Part model, mm, in its own coordinate system. Face numbers are marked on the shaded views. A direction names the side the tool comes from. Give positions to 0.01 mm unless a question says otherwise; leave off trailing zeros. Order: outer loops, then holes, each group sorted by start corner. A loop starts at its lowest first (then second) coordinate and runs counter-clockwise, first axis right, second up. Notation, with made-up numbers: M 46,-36 L 65,-36 A11 cw 65,-28 Z; hole C 67,79.5 d10. An arc over 180 degrees is marked long. Write each question's results on one line, items separated by ' | '. Start each with the question number.
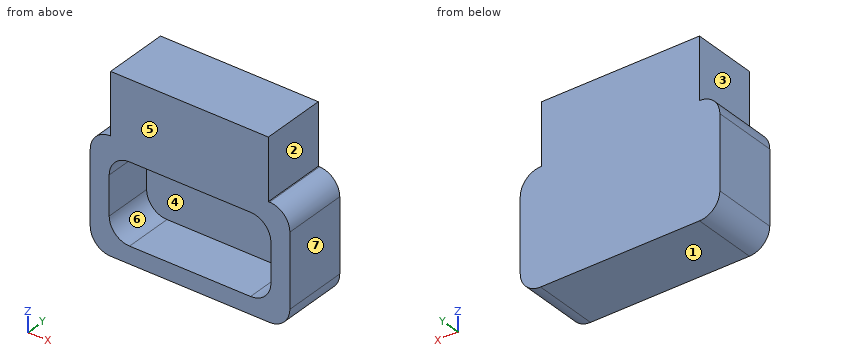
from build123d import *

# Parameters (mm, degrees)
F1_DEPTH = 19.05
F2_DEPTH = 5.08
F0_W     = 49.223448
F0_H     = 19.05
F3_DEPTH = 20.32


with BuildPart() as f1:
    # F0 (on Front) → F1 (new body)
    with BuildSketch(Plane.XZ):
        with BuildLine():
            Line((24.436552, 17.736208), (-24.786896, 17.736208))
            ThreePointArc((-24.786896, 17.736208), (-29.277025, 15.876336), (-31.136896, 11.386208))
            Line((-31.136896, 11.386208), (-31.136896, -11.386208))
            ThreePointArc((-31.136896, -11.386208), (-29.277025, -15.876336), (-24.786896, -17.736208))
            Line((-24.786896, -17.736208), (24.786896, -17.736208))
            ThreePointArc((24.786896, -17.736208), (29.277025, -15.876336), (31.136896, -11.386208))
            Line((31.136896, -11.386208), (31.136896, 11.386208))
            ThreePointArc((31.136896, 11.386208), (29.277025, 15.876336), (24.786896, 17.736208))
            Line((24.786896, 17.736208), (24.436552, 17.736208))
        make_face()
        with BuildLine():
            ThreePointArc((-25.224827, 6.065345), (-23.364955, 10.555473), (-18.874827, 12.415345))
            Line((-18.874827, 12.415345), (18.874827, 12.415345))
            ThreePointArc((18.874827, 12.415345), (23.364955, 10.555473), (25.224827, 6.065345))
            Line((25.224827, 6.065345), (25.224827, -6.065345))
            ThreePointArc((25.224827, -6.065345), (23.364955, -10.555473), (18.874827, -12.415345))
            Line((18.874827, -12.415345), (-18.874827, -12.415345))
            ThreePointArc((-18.874827, -12.415345), (-23.364955, -10.555473), (-25.224827, -6.065345))
            Line((-25.224827, -6.065345), (-25.224827, 6.065345))
        make_face(mode=Mode.SUBTRACT)
    extrude(amount=F1_DEPTH)

    # F0 (on Front) → F2 (join)
    with BuildSketch(Plane.XZ):
        with BuildLine():
            Line((18.874827, 12.415345), (-18.874827, 12.415345))
            ThreePointArc((-18.874827, 12.415345), (-23.364955, 10.555473), (-25.224827, 6.065345))
            Line((-25.224827, 6.065345), (-25.224827, -6.065345))
            ThreePointArc((-25.224827, -6.065345), (-23.364955, -10.555473), (-18.874827, -12.415345))
            Line((-18.874827, -12.415345), (18.874827, -12.415345))
            ThreePointArc((18.874827, -12.415345), (23.364955, -10.555473), (25.224827, -6.065345))
            Line((25.224827, -6.065345), (25.224827, 6.065345))
            ThreePointArc((25.224827, 6.065345), (23.364955, 10.555473), (18.874827, 12.415345))
        make_face()
    extrude(amount=F2_DEPTH)

    # F0 (on Front) → F3 (join)
    with BuildSketch(Plane.XZ):
        with Locations((-0.175172, 27.261208)):
            Rectangle(F0_W, F0_H)
        with BuildLine():
            Line((24.436552, 17.736208), (-24.786896, 17.736208))
            ThreePointArc((-24.786896, 17.736208), (-29.277025, 15.876336), (-31.136896, 11.386208))
            Line((-31.136896, 11.386208), (-31.136896, -11.386208))
            ThreePointArc((-31.136896, -11.386208), (-29.277025, -15.876336), (-24.786896, -17.736208))
            Line((-24.786896, -17.736208), (24.786896, -17.736208))
            ThreePointArc((24.786896, -17.736208), (29.277025, -15.876336), (31.136896, -11.386208))
            Line((31.136896, -11.386208), (31.136896, 11.386208))
            ThreePointArc((31.136896, 11.386208), (29.277025, 15.876336), (24.786896, 17.736208))
            Line((24.786896, 17.736208), (24.436552, 17.736208))
        make_face()
        with BuildLine():
            ThreePointArc((-25.224827, 6.065345), (-23.364955, 10.555473), (-18.874827, 12.415345))
            Line((-18.874827, 12.415345), (18.874827, 12.415345))
            ThreePointArc((18.874827, 12.415345), (23.364955, 10.555473), (25.224827, 6.065345))
            Line((25.224827, 6.065345), (25.224827, -6.065345))
            ThreePointArc((25.224827, -6.065345), (23.364955, -10.555473), (18.874827, -12.415345))
            Line((18.874827, -12.415345), (-18.874827, -12.415345))
            ThreePointArc((-18.874827, -12.415345), (-23.364955, -10.555473), (-25.224827, -6.065345))
            Line((-25.224827, -6.065345), (-25.224827, 6.065345))
        make_face(mode=Mode.SUBTRACT)
    extrude(amount=F3_DEPTH)


solid = f1.part
(1) Drop flat-ended pins along their axis: P1, Ø8, axis at x = 11.5, z = -7.5, coming from the -Y side; P2, Ø2, axis at y = -16.5, z = 19, coming from the -X side. Give the stop position or say it passes through.
(2) Tool access for the marked faces 1, 2, 3 and 4: list every direction of +Z, -Z, +X, -X, +Y, -Y with a clear straight run to the whole face (end or side of a thin tool).
(3) Probe L1, parallel to X at y = -11, z = -0.5; L2, parallel to Z at x = 6.5, y = -6.5; L3, parallel to Y at x = 24, z = 2. List the from-to ranges inside material, lowest first.
(4) Saw through at D-D on y = -3.75. Give the cut face in (x, z), plus the area to 3 significant figures.
(5) Saw through at A-A on y = -15.75. Give the cut face in (x, z).
(6) Saw through at B-B on x = -11.5. Give the cut face in (y, z).
(7) Saw through at C-C on z = -0.5. Give the cut face in (x, y).
(8) Pull direction X, two halves, no side cores. Call the marked faces 5, 6 and 7: +X half, -X half, draft (parallel to the pull), parting line (faces both ways), or undercut.
Taken from the geometry:
1) P1: stops at y = -5.08 | P2: stops at x = -24.79
2) face 1: -Z, +X, -X, +Y, -Y | face 2: +Z, +X, +Y, -Y | face 3: +Z, -X, +Y, -Y | face 4: -Y
3) L1: x = -31.14 to -25.22, 25.22 to 31.14 | L2: z = -17.74 to -12.42, 12.42 to 36.79 | L3: y = -5.08 to 0
4) outline: M -31.14,-11.39 A6.35 ccw -24.79,-17.74 L 24.79,-17.74 A6.35 ccw 31.14,-11.39 L 31.14,11.39 A6.35 ccw 24.79,17.74 L 24.44,17.74 L 24.44,36.79 L -24.79,36.79 L -24.79,17.74 A6.35 ccw -31.14,11.39 Z | area: 3,110 mm²
5) outline: M -31.14,-11.39 A6.35 ccw -24.79,-17.74 L 24.79,-17.74 A6.35 ccw 31.14,-11.39 L 31.14,11.39 A6.35 ccw 24.79,17.74 L 24.44,17.74 L 24.44,36.79 L -24.79,36.79 L -24.79,17.74 A6.35 ccw -31.14,11.39 Z; hole M -25.22,-6.07 A6.35 ccw -18.87,-12.42 L 18.87,-12.42 A6.35 ccw 25.22,-6.07 L 25.22,6.07 A6.35 ccw 18.87,12.42 L -18.87,12.42 A6.35 ccw -25.22,6.07 Z
6) outline: M -20.32,-17.74 L 0,-17.74 L 0,36.79 L -20.32,36.79 L -20.32,12.42 L -5.08,12.42 L -5.08,-12.42 L -20.32,-12.42 Z
7) outline: M -31.14,-20.32 L -25.22,-20.32 L -25.22,-5.08 L 25.22,-5.08 L 25.22,-20.32 L 31.14,-20.32 L 31.14,0 L -31.14,0 Z
8) face 5: draft | face 6: undercut | face 7: +X half
